Read the model definition and answer for the solid it produces. Units are mm, in the model's axes. Give positions to 0.01 mm unless a question says otherwise; leave off trailing zeros. Loops run counter-clockwise (first coordinate to the right, second up) from the corner with the lowest first, then second, coordinate; pieces in that order, holes last.
(1) Find section C-C, the plane z = 9. Write down the section's boundary in (x, y) (3 decimals), then the cut area to 3 significant figures.
(2) Find section B-B, the plane x = 11.5. Write down the section's boundary in (y, z), then the cut area to 3 significant figures.
(3) Find section D-D, the plane x = 0. State how many separate pieces and enclosed holes the cut face has, then the cut area to 3 significant figures.
(4) This flat-tipped pin is pushed along its axis until it touches: P1, Ø4, axis at x = 0, y = 13.335, coming from the -Z side. Where does it stop, or does it pass through?
(5) Straight lines are drawn through the part: probe 1 along Y at (x, z) = (0, 16); probe 2 along Z at (x, y) = (-1, 1.5). For each, find the intervals that lie inside material, in ascending order.
(6) Find section A-A, the plane y = 42.5. Write down the section's boundary in (x, z).
```python
from build123d import *

# Parameters (mm, degrees)
SKETCH1_W             = 20.828
SKETCH1_H             = 20.828
BOSS_EXTRUDE1_DEPTH   = 50.8
SKETCH1_W_2           = 39.116
SKETCH1_H_2           = 39.116
SKETCH1_W_3           = 26.416
SKETCH1_H_3           = 26.416
BOSS_EXTRUDE1_2_DEPTH = 50.8
SKETCH2_R             = 2.286
CUT_EXTRUDE1_DEPTH    = 40.116
SKETCH1_2_W           = 39.116
SKETCH1_2_H           = 39.116
SKETCH1_2_W_2         = 26.416
SKETCH1_2_H_2         = 26.416
SKETCH1_2_W_3         = 20.828
SKETCH1_2_H_3         = 20.828
BOSS_EXTRUDE2_DEPTH   = 6.35
FILLET1_R             = 2.54


with BuildPart() as part:
    # Sketch1 → Boss-Extrude1 (new body)
    with BuildSketch(Plane(origin=(0, 0, 0), x_dir=(1, 0, 0), z_dir=(0, 1, 0))):
        Rectangle(SKETCH1_W, SKETCH1_H)
    extrude(amount=BOSS_EXTRUDE1_DEPTH)


with BuildPart() as body_2:
    # Sketch1 → Boss-Extrude1 2 (new body)
    with BuildSketch(Plane(origin=(0, 0, 0), x_dir=(1, 0, 0), z_dir=(0, 1, 0))):
        Rectangle(SKETCH1_W_2, SKETCH1_H_2)
        Rectangle(SKETCH1_W_3, SKETCH1_H_3, mode=Mode.SUBTRACT)
    extrude(amount=BOSS_EXTRUDE1_2_DEPTH)


with BuildPart() as cut_extrude1_tool:
    # Sketch2 → Cut-Extrude1 (new body, through all)
    with BuildSketch(Plane.XY.offset(19.558)):
        with Locations((0, 13.335)):
            Circle(SKETCH2_R)
        with Locations((0, 38.735)):
            Circle(SKETCH2_R)
    extrude(amount=-CUT_EXTRUDE1_DEPTH)


with BuildPart() as part_1:
    add(part.part)

    # Cut-Extrude1: cut by cut_extrude1_tool
    add(cut_extrude1_tool.part, mode=Mode.SUBTRACT)



with BuildPart() as body_2_1:
    add(body_2.part)

    # Cut-Extrude1: cut by cut_extrude1_tool
    add(cut_extrude1_tool.part, mode=Mode.SUBTRACT)


with BuildPart() as part_2:
    add(part_1.part)

    add(body_2_1.part)  # Boss-Extrude2 merges body 2
    # Sketch1_2 → Boss-Extrude2 (add)
    with BuildSketch(Plane(origin=(0, 0, 0), x_dir=(1, 0, 0), z_dir=(0, 1, 0))):
        Rectangle(SKETCH1_2_W, SKETCH1_2_H)
        Rectangle(SKETCH1_2_W_2, SKETCH1_2_H_2, mode=Mode.SUBTRACT)
        Rectangle(SKETCH1_2_W_2, SKETCH1_2_H_2)
        Rectangle(SKETCH1_2_W_3, SKETCH1_2_H_3, mode=Mode.SUBTRACT)
        Rectangle(SKETCH1_2_W_3, SKETCH1_2_H_3)
    extrude(amount=-BOSS_EXTRUDE2_DEPTH)

    # Fillet1
    fillet1_edges = [part_2.edges().sort_by_distance(p)[0] for p in [
        (-19.558, 22.225, 19.558),
        (-19.558, 22.225, -19.558),
        (19.558, 22.225, -19.558),
        (19.558, 22.225, 19.558),
        (10.414, 25.4, -10.414),
        (10.414, 25.4, 10.414),
        (-10.414, 25.4, 10.414),
        (-10.414, 25.4, -10.414),
    ]]
    fillet(fillet1_edges, radius=FILLET1_R)


solid = part_2.part
```
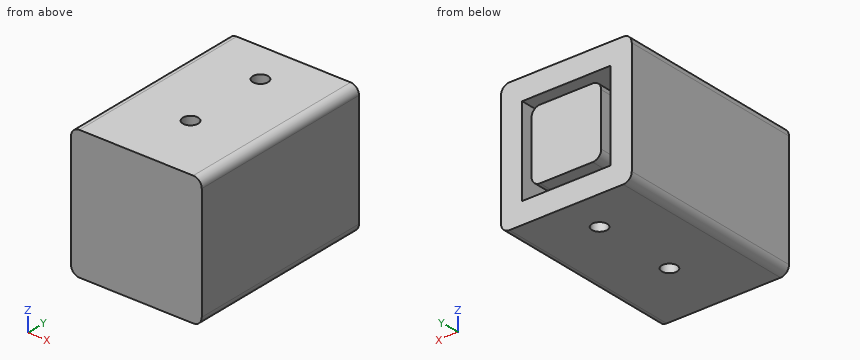
Entries:
1. outline: (-19.558, -6.35) - (19.558, -6.35) - (19.558, 50.8) - (13.208, 50.8) - (13.208, 0) - (10.151, 0) - (10.151, 50.8) - (-10.151, 50.8) - (-10.151, 0) - (-13.208, 0) - (-13.208, 50.8) - (-19.558, 50.8) - close; hole circle Ø4.572 at (0, 13.335); hole circle Ø4.572 at (0, 38.735)
1. area: 1,890 mm2
2. outline: (-6.35, -19.56) - (50.8, -19.56) - (50.8, -13.21) - (0, -13.21) - (0, 13.21) - (50.8, 13.21) - (50.8, 19.56) - (-6.35, 19.56) - close
2. area: 894 mm2
3. separate pieces: 7
3. enclosed holes: 0
3. area: 1,650 mm2
4. P1: passes through
5. probe 1: y = -6.35 to 11.05, 15.62 to 36.45, 41.02 to 50.8
5. probe 2: z = -19.56 to -13.21, -10.41 to 10.41, 13.21 to 19.56
6. outline: (-19.56, -17.02) arc R2.54 ccw to (-17.02, -19.56) - (17.02, -19.56) arc R2.54 ccw to (19.56, -17.02) - (19.56, 17.02) arc R2.54 ccw to (17.02, 19.56) - (-17.02, 19.56) arc R2.54 ccw to (-19.56, 17.02) - close; (-10.41, -7.87) arc R2.54 ccw to (-7.87, -10.41) - (7.87, -10.41) arc R2.54 ccw to (10.41, -7.87) - (10.41, 7.87) arc R2.54 ccw to (7.87, 10.41) - (-7.87, 10.41) arc R2.54 ccw to (-10.41, 7.87) - close; hole (-13.21, -13.21) - (13.21, -13.21) - (13.21, 13.21) - (-13.21, 13.21) - close
